The figure shows three views and two pictorial views of one solid part (mm, origin at its lowest corner). Answer the questions. A direction names the side the tool comes from. Round coordinates to 2 decimals unless told otherwise and drop trailing zeros. Write each loop counter-clockwise with the first axis right and the second up, starting at its lowest first coordinate (ties: lowest second). Pieces come first, ordered by that corner, then holes.
Item 1: Find section C-C on z = 12.7. Give the vertices of the cut face in (x, y) (3 decimals), then the cut area to 3 significant figures.
Item 2: Find section D-D on x = 9.5. Give the vertices of the cut face in (y, z), then the cut area to 3 significant figures.
Item 3: Find section A-A on y = 55. Give the vertices of the cut face in (x, z) (3 decimals), then the cut area to 3 significant figures.
Item 4: Each of these flat-tipped pins is pushed along its axis until it touches: pin 1 (5 mm diameter, centred on x = 43, z = 32.5, fed in from +Y); pin 2 (3 mm diameter, centred on x = 32, z = 11.5, fed in from -Y); pin 3 (1.9 mm diameter, centred on x = 19, z = 31, fed in from +Y). Where does it stop, or does it pass through?
Item 5: Find section B-B on x = 44.45. Give the vertices of the cut face in (y, z) (3 decimals), then the cut area to 3 significant figures.
Item 6: Find the intervals of material crossed by probe 1 along Z at (x, y) = (31.75, 3.25) (3 decimals); probe 2 along X at (y, z) = (60, 31); probe 3 along X at (y, z) = (61, 34), in increasing order.
Item 7: A tool of negligible diameter and unlimited length cuts with its end or side. For the marked faces 1 and 2, from which of +Z, -Z, +X, -X, +Y, -Y can it reach the whole face along a straight path? Write none if from no direction.
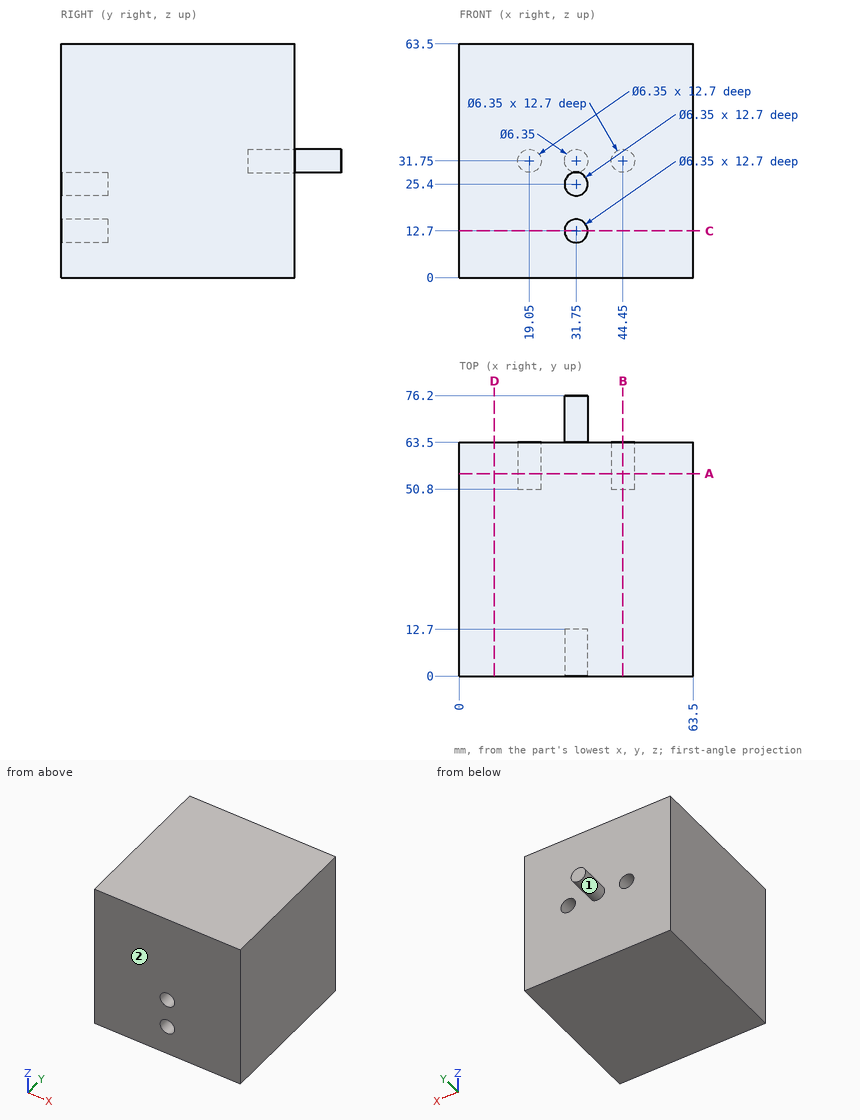
Check values:
1. outline: (0, 0) - (28.575, 0) - (28.575, 12.7) - (34.925, 12.7) - (34.925, 0) - (63.5, 0) - (63.5, 63.5) - (0, 63.5) - close
1. area: 3,950 mm2
2. outline: (0, 0) - (63.5, 0) - (63.5, 63.5) - (0, 63.5) - close
2. area: 4,030 mm2
3. outline: (0, 0) - (63.5, 0) - (63.5, 63.5) - (0, 63.5) - close; hole circle Ø6.35 at (19.05, 31.75); hole circle Ø6.35 at (44.45, 31.75)
3. area: 3,970 mm2
4. pin 1: stops at y = 63.5
4. pin 2: stops at y = 12.7
4. pin 3: stops at y = 50.8
5. outline: (0, 0) - (63.5, 0) - (63.5, 28.575) - (50.8, 28.575) - (50.8, 34.925) - (63.5, 34.925) - (63.5, 63.5) - (0, 63.5) - close
5. area: 3,950 mm2
6. probe 1: z = 0 to 9.525, 15.875 to 22.225, 28.575 to 63.5
6. probe 2: x = 0 to 15.96, 22.14 to 41.36, 47.54 to 63.5
6. probe 3: x = 0 to 16.81, 21.29 to 42.21, 46.69 to 63.5
7. face 1: +Y
7. face 2: +Z, -Z, +X, -X, -Y
